Build history of the part. All positions in model axes, mm. Face numbers are marked on the shaded views. Coordinates: 2 decimals unless noted, no trailing zeros. Loops run counter-clockwise (first coordinate to the right, second up) from the corner with the lowest first, then second, coordinate; pieces in that order, holes last.
Item 1: Cut at D-D (z = -7.5). List the corners of the cut face in (x, y), and give its area (3 significant figures).
Item 2: Cut at C-C (z = 10). List the corners of the cut face in (x, y).
Item 3: Cut at A-A (y = 0). List the corners of the cut face in (x, z), and give its area (3 significant figures).
Item 4: Mould opens along X. For the marked faces 1, 2 and 3 say: released by +X, released by -X, zero draft, split by the parting line, or undercut.
Item 5: Drill centre lines: line 1 along Z through (x, y) = (-15, 0); line 2 along X through (y, z) = (0, -4); line 3 along X through (y, z) = (16, 16). Where is each one in solid material? Low to high.
Item 6: Cut at B-B (x = 0). List the corners of the cut face in (y, z).
Item 7: Flat gauge pins, fed straight in: pin 1 (3 mm diameter, centred on y = 2, z = 2, fed in from -X); pin 2 (4 mm diameter, centred on x = -5.5, z = -3, fed in from +Y); pin 3 (2.5 mm diameter, centred on x = 0, z = -7.5, fed in from -Y); pin 4 (15 mm diameter, centred on x = 0, y = 0, fed in from +Z). Where does each tip first touch, or does it go through?
from build123d import *

# Parameters (mm, degrees)
SKETCH_1_R                  = 20
SKETCH_1_R_2                = 9.5
EXTRUDE_1_DEPTH             = 22.5
SKETCH_3_W                  = 6
SKETCH_3_H                  = 6
CUT_EXTRUDE_2_DEPTH         = 54.150729064
HOLE_WIZARD_M5_1_AT_2_COUNT = 2
HOLE_WIZARD_M5_1_AT_2_PITCH = 24
PATTERN_CIRCULAR_1_COUNT    = 2
PATTERN_CIRCULAR_1_ANGLE    = 90
CHAMFER_1_SIZE              = 1


with BuildPart() as part:
    # 草图1 → 凸台-拉伸1 (new, symmetric)
    with BuildSketch(Plane.XY):
        with Locations(Location((0, 0, 0), (0, 0, 180))):
            Circle(SKETCH_1_R)
        with Locations(Location((0, 0, 0), (0, 0, 180))):
            Circle(SKETCH_1_R_2, mode=Mode.SUBTRACT)
    extrude(amount=EXTRUDE_1_DEPTH, both=True)

    # 草图3 → 切除-拉伸2 (cut, through all)
    with BuildSketch(Plane(origin=(0, 0, -22.5), x_dir=(-1, 0, 0), z_dir=(0, 0, -1))):
        with Locations((0, 9.5)):
            Rectangle(SKETCH_3_W, SKETCH_3_H)
    extrude(amount=-CUT_EXTRUDE_2_DEPTH, mode=Mode.SUBTRACT)

    # 草图4 → M5 螺纹孔1 (revolve, cut)
    with BuildSketch(Plane(origin=(-20, 0, 16.5), x_dir=(0, 0, 1), z_dir=(0, 1, 0))):
        Polygon((0, 0), (0, 20.2618073), (2.1, 19), (2.1, 0), align=None)
    hole_wizard_m5_1 = revolve(axis=Axis((-26.35, 0, 16.5), (1, 0, 0)), mode=Mode.SUBTRACT)

    # M5 螺纹孔1 at 2: M5 螺纹孔1 ×2
    with Locations(*[(0, 0, -i * HOLE_WIZARD_M5_1_AT_2_PITCH) for i in range(1, HOLE_WIZARD_M5_1_AT_2_COUNT)]):
        add(hole_wizard_m5_1, mode=Mode.SUBTRACT)

    # 阵列(圆周)1: M5 螺纹孔1 ×2 about axis
    pattern_circular_1_axis = Axis((0, 0, 22.5), (0, 0, -1))
    for i in range(1, PATTERN_CIRCULAR_1_COUNT):
        add(hole_wizard_m5_1.rotate(pattern_circular_1_axis, i * PATTERN_CIRCULAR_1_ANGLE / (PATTERN_CIRCULAR_1_COUNT - 1)), mode=Mode.SUBTRACT)

    # 阵列(圆周)1 copy 1 sketch → 阵列(圆周)1 copy 1 (revolve, cut)
    with BuildSketch(Plane(origin=(0, 20, -7.5), x_dir=(0, 0, 1), z_dir=(1, 0, 0))):
        Polygon((0, 0), (0, 20.2618073), (2.1, 19), (2.1, 0), align=None)
    revolve(axis=Axis((0, 26.35, -7.5), (0, -1, 0)), mode=Mode.SUBTRACT)

    # 倒角1
    chamfer_1_edges = [part.edges().sort_by_distance(p)[0] for p in [
        (20, 0, -22.5),
        (20, 0, 22.5),
    ]]
    chamfer(chamfer_1_edges, length=CHAMFER_1_SIZE)


solid = part.part
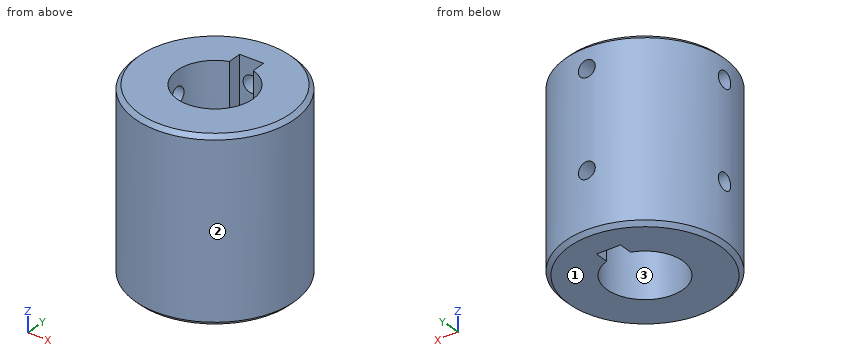
Filled sheet:
1. outline: (-19.89, -2.1) arc R20 ccw (long way) to (2.1, 19.89) - (2.1, 12.5) - (3, 12.5) - (3, 9.01) arc R9.5 cw (long way) to (-9.26, -2.1) - close; (-19.89, 2.1) - (-9.26, 2.1) arc R9.5 cw to (-3, 9.01) - (-3, 12.5) - (-2.1, 12.5) - (-2.1, 19.89) arc R20 ccw to start
1. area: 879 mm2
2. outline: circle Ø40 at (0, 0); hole (-3, 9.01) arc R9.5 ccw (long way) to (3, 9.01) - (3, 12.5) - (-3, 12.5) - close
3. outline: (-20, -21.5) - (-19, -22.5) - (-9.5, -22.5) - (-9.5, -9.6) - (-20, -9.6) - close; (-20, -5.4) - (-9.5, -5.4) - (-9.5, 14.4) - (-20, 14.4) - close; (-20, 18.6) - (-9.5, 18.6) - (-9.5, 22.5) - (-19, 22.5) - (-20, 21.5) - close; (9.5, -22.5) - (19, -22.5) - (20, -21.5) - (20, 21.5) - (19, 22.5) - (9.5, 22.5) - close
3. area: 855 mm2
4. face 1: zero draft
4. face 2: split by the parting line
4. face 3: undercut
5. line 1: z = -22.5 to -9.6, -5.4 to 14.4, 18.6 to 22.5
5. line 2: x = -20 to -9.5, 9.5 to 20
5. line 3: x = -12 to -2.04, 2.04 to 12
6. outline: (-20, -21.5) - (-19, -22.5) - (-9.5, -22.5) - (-9.5, 22.5) - (-19, 22.5) - (-20, 21.5) - close; (12.5, -22.5) - (19, -22.5) - (20, -21.5) - (20, -9.6) - (12.5, -9.6) - close; (12.5, -5.4) - (20, -5.4) - (20, 14.4) - (12.5, 14.4) - close; (12.5, 18.6) - (20, 18.6) - (20, 21.5) - (19, 22.5) - (12.5, 22.5) - close
7. pin 1: stops at x = -19.99
7. pin 2: stops at y = 19.69
7. pin 3: stops at y = -20
7. pin 4: passes through
